Autodesk Inventor part; units mm, degrees
ref_plane "YZ Plane" through (0, 0, 0) normal (1, 0, 0) x (0, 1, 0)
ref_plane "XZ Plane" through (0, 0, 0) normal (0, 1, 0) x (-1, 0, 0)
ref_plane "XY Plane" through (0, 0, 0) normal (0, 0, 1) x (1, 0, 0)
sketch "Sketch1" plane through (0, 0, 0) normal (0, 0, 1) x (1, 0, 0)
  line L0 (4, 3.875) -> (-4, 3.875)
  line L1 (-4, 3.875) -> (-4, -3.875)
  line L2 (-4, -3.875) -> (4, -3.875)
  line L3 (4, -3.875) -> (4, 3.875)
  line L4 (4, 3.875) -> (-4, -3.875) construction
  line L5 (-4, 3.875) -> (4, -3.875) construction
  line L6 (4, 3.875) -> (9.5, 3.875)
  line L7 (-4, 3.875) -> (-9.5, 3.875)
  line L8 (4, -3.875) -> (9.5, 3.875)
  line L9 (-4, -3.875) -> (-9.5, 3.875)
  point P0 (0, 0)
  point P1 (0, 3.875)
  dimension "d0" = 8
  dimension "d1" = 7.75
  dimension "d2" = 9.5
  dimension "d3" = 9.5
extrude "Extrusion1" add sketch "Sketch1" along normal blind 25
sketch "Sketch2" plane through (-9.5, 3.875, 0) normal (0, 1, 0) x (1, 0, 0)
  line L0 (0, 0) -> (5.5, 0)
  line L1 (5.5, -25) -> (13.5, -25)
  line L2 (5.5, 0) -> (5.5, -25)
  line L3 (5.5, -25) -> (13.5, -25)
  line L4 (13.5, 0) -> (19, 0)
  line L5 (13.5, -25) -> (13.5, 0)
  line L6 (5.5, 0) -> (13.5, 0)
  line L7 (13.5, 0) -> (5.5, 0)
  point P0 (9.5, 0)
  dimension "d6" = 8
extrude "Extrusion2" add sketch "Sketch2" along normal blind 5
sketch "Sketch3" plane through (0, 0, 25) normal (0, 0, 1) x (1, 0, 0)
  line L0 (0, 0) -> (14.2258, 0)
  line L1 (-4, -3.875) -> (4, -3.875)
  line L2 (4, -3.875) -> (9.5, 3.875)
  line L3 (4, -3.875) -> (9.5, 3.875)
  line L4 (9.5, 3.875) -> (4, 3.875)
  line L5 (4, 3.875) -> (4, 8.875)
  line L6 (4, 3.875) -> (4, 8.875)
  line L7 (-4, 3.875) -> (-4, 8.875)
  line L8 (4, 8.875) -> (-4, 8.875)
  line L9 (-4, 8.875) -> (-4, 3.875)
  line L10 (-4, 3.875) -> (-9.5, 3.875)
  line L11 (-4, 3.875) -> (-9.5, 3.875)
  line L12 (-9.5, 3.875) -> (-4, -3.875)
  line L13 (42.75, -3.875) -> (48.25, 3.875)
  line L14 (48.25, 3.875) -> (42.75, 3.875)
  line L15 (42.75, 3.875) -> (42.75, 8.875)
  line L16 (42.75, 8.875) -> (34.75, 8.875)
  line L17 (34.75, 8.875) -> (34.75, 3.875)
  line L18 (34.75, 3.875) -> (29.25, 3.875)
  line L19 (29.25, 3.875) -> (34.75, -3.875)
  line L20 (34.75, -3.875) -> (42.75, -3.875)
  line L21 (34.75, 8.875) -> (42.75, 8.875)
  line L22 (42.75, 8.875) -> (42.75, 8.975)
  line L23 (42.75, 8.975) -> (34.75, 8.975)
  line L24 (34.75, 8.975) -> (34.75, 8.875)
  line L25 (4, 8.875) -> (-4, 8.875)
  line L26 (-4, 8.875) -> (-4, 8.975)
  line L27 (-4, 8.975) -> (4, 8.975)
  line L28 (4, 8.975) -> (4, 8.875)
  line L29 (-4, 8.975) -> (42.75, 8.975)
  line L30 (42.75, 8.975) -> (42.75, 10.675)
  line L31 (42.75, 10.675) -> (-4, 10.675)
  line L32 (-4, 10.675) -> (-4, 8.975)
  point P0 (6.75, 0)
  point P1 (38.75, 0)
  point P2 (52.9758, 0)
  point P3 (45.5, 0)
  dimension "d9" = 6.75
  dimension "d12" = 38.75
  dimension "d19" = 1.7
  dimension "d22" = 0.1
extrude "Extrusion3" add sketch "Sketch3" against normal blind 25 contours L26 L27 L28 L8 | L23 L22 L16 L24 | L16 L15 L14 L13 L20 L19 L18 L17
extrude "Extrusion4" add sketch "Sketch3" against normal blind 25 contours L32 L31 L30 L23 L29 L27
sketch "Sketch4" plane through (0, 0, 25) normal (0, 0, 1) x (1, 0, 0)
  line L0 (42.75, 10.675) -> (-4, 10.675)
  line L1 (-4, 10.675) -> (42.75, 10.675)
  line L2 (42.75, 10.675) -> (42.75, 92.475)
  line L3 (42.75, 92.475) -> (-4, 92.475)
  line L4 (-4, 92.475) -> (-4, 10.675)
  line L5 (-4, 10.675) -> (11, 10.675)
  line L6 (11, 10.675) -> (11, 92.475)
  line L7 (11, 92.475) -> (-4, 92.475)
  line L8 (-4, 92.475) -> (-4, 10.675)
  line L9 (78.9241, 46.475) -> (-27.5343, 46.475)
  line L10 (-27.5343, 46.475) -> (-27.5343, 66.675)
  line L11 (-27.5343, 66.675) -> (78.9241, 66.675)
  line L12 (78.9241, 66.675) -> (78.9241, 46.475)
  line L13 (4, 8.975) -> (34.75, 8.975)
  line L14 (-36.8215, 45.475) -> (107.9586, 45.475)
  line L15 (107.9586, 45.475) -> (107.9586, 29.475)
  line L16 (107.9586, 29.475) -> (-36.8215, 29.475)
  line L17 (-36.8215, 29.475) -> (-36.8215, 45.475)
  line L18 (-39.8107, 67.675) -> (114.95, 67.675)
  line L19 (114.95, 67.675) -> (114.95, 83.675)
  line L20 (114.95, 83.675) -> (-39.8107, 83.675)
  line L21 (-39.8107, 83.675) -> (-39.8107, 67.675)
  point P0 (0, 0)
  dimension "d23" = 81.8
  dimension "d24" = 15
  dimension "d25" = 37.5
  dimension "d26" = 20.2
  dimension "d27" = 16
  dimension "d28" = 18.8
  dimension "d29" = 16
  dimension "d30" = 1
  dimension "d31" = 1
  dimension "d36" = 8.8
  dimension "d37" = 47
extrude "Extrusion5" add sketch "Sketch4" against normal blind 25 contours L0 L4 L16 L6 | L16 L4 L14 L6 | L14 L4 L9 L6 | L9 L4 L11 L6 | L11 L4 L18 L6 | L18 L4 L20 L6 | L20 L4 L3 L6
sketch "Sketch5" plane through (0, 0, 25) normal (0, 0, 1) x (1, 0, 0)
  line L0 (11, 92.475) -> (11, 10.675)
  line L1 (42.75, 10.675) -> (42.75, 3.875)
  arc A0 (11, 16.49) -> (42.75, 10.675) centre (50.7681, 144.0402) ccw
  line L2 (11, 16.49) -> (11, 10.675)
  line L3 (11, 10.675) -> (42.75, 10.675)
  line L4 (42.75, 10.675) -> (11, 10.675)
  line L5 (34.75, 8.975) -> (4, 8.975)
  point P0 (0, 0)
extrude "Extrusion6" add sketch "Sketch5" against normal blind 25
sketch "Sketch6" plane through (-4, 3.875, 0) normal (-1, 0, 0) x (0, 0, 1)
  line L0 (25, 88.6) -> (0, 88.6)
  line L1 (25, 0) -> (25, 88.6)
  circle A0 centre (12.5, 71.8) radius 8.5
  circle A1 centre (12.5, 33.6) radius 8.5
  point P0 (0, -3.875)
  dimension "d38" = 16.8
  dimension "d39" = 12.5
  dimension "d40" = 17
  dimension "d41" = 55
  dimension "d42" = 17
extrude "Extrusion7" cut sketch "Sketch6" against normal blind 25
sketch "Sketch7" plane through (0, 0, 25) normal (0, 0, 1) x (1, 0, 0)
  line L0 (11, 16.49) -> (11, 92.475)
  line L1 (11, 92.475) -> (-4, 92.475)
  point P0 (0, 0)
  point P1 (3.5, 75.675)
  point P2 (3.5, 92.475)
  point P3 (3.5, 37.475)
  dimension "d45" = 7.5
  dimension "d46" = 16.8
  dimension "d47" = 55
hole "Hole1" at (3.5, 37.475, 25) at (3.5, 75.675, 25) direction (0, 0, -1) diameter 4 end through all
CAD build for the part. Positions are in the model's coordinates, mm. A direction names the side the tool comes from. Give positions to 0.01 mm unless a question says otherwise; leave off trailing zeros. Order: outer loops, then holes, each group sorted by start corner. A loop starts at its lowest first (then second) coordinate and runs counter-clockwise, first axis right, second up.
(1) Saw through at D-D, the plane y = 45. Give the cut face in (x, z).
(2) Saw through at C-C, the plane y = 81.5. Give the cut face in (x, z).
(3) Mould opens along Z. For faces 1 (the flat face through (9, 41, 25)), 2 (the cylindrical face through (3.395, 40.028, 20.607)), 3 (the flat face through (39, -3.875, 13)), 4 (the flat face through (9, 41, 0)) say: released by +Z, released by -Z, zero draft, split by the parting line, or undercut.
(4) Saw through at A-A, the plane z = 2.25. Give the cut face in (x, y) (3 decimals).
(5) Drill centre lines: L1, parallel to Y at x = 0, z = 12.5 (3 decimals); L2, parallel to Y at x = 3.5, z = 24.1 (3 decimals); L3, parallel to X at y = 5.5, z = 6.5. Where is each one in solid material? Low to high.
(6) Flat gauge pins, fed straight in: pin 1 (1.5 mm diameter, centred on y = 7.5, z = 14.5, fed in from -X); pin 2 (3 mm diameter, centred on x = 44.5, z = 13.5, fed in from +Y) (3 decimals); pin 3 (10 mm diameter, centred on y = 30.5, z = 19, fed in from +X); pin 4 (2.5 mm diameter, centred on x = 3.5, y = 37.475, fed in from -Z). Where does each tip first touch, or does it go through?
(7) Saw through at B-B, the plane z = 12.5. Give the cut face in (x, y) (3 decimals), then the cut area to 3 significant figures.
(8) Tool access for faces 5 (the flat face through (45.461, -0.054, 12.675)), 6 (the flat face through (-4, 49, 13)), 7 (the flat face through (6.711, -0.054, 12.325)), 8 (the flat face through (46, 3.875, 13)), 9 (the flat face through (32, 3.875, 13)): list every direction of +Z, -Z, +X, -X, +Y, -Y with a clear straight run to the whole face (end or side of a thin tool).
Results found:
1. outline: (-4, 0) - (11, 0) - (11, 8.55) - (-4, 8.55) - close; (-4, 16.45) - (11, 16.45) - (11, 25) - (-4, 25) - close
2. outline: (-4, 0) - (11, 0) - (11, 6.31) - (-4, 6.31) - close; (-4, 18.69) - (11, 18.69) - (11, 25) - (-4, 25) - close
3. face 1: released by +Z
3. face 2: undercut
3. face 3: zero draft
3. face 4: released by -Z
4. outline: (-9.5, 3.875) - (-4, -3.875) - (4, -3.875) - (9.5, 3.875) - (4, 3.875) - (4, 8.975) - (34.75, 8.975) - (34.75, 3.875) - (29.25, 3.875) - (34.75, -3.875) - (42.75, -3.875) - (48.25, 3.875) - (42.75, 3.875) - (42.75, 10.675) arc R133.609 cw to (11, 16.49) - (11, 92.475) - (-4, 92.475) - (-4, 3.875) - close; hole circle Ø4 at (3.5, 37.475); hole circle Ø4 at (3.5, 75.675)
5. L1: y = -3.875 to 28.975, 45.975 to 67.175, 84.175 to 92.475
5. L2: y = -3.875 to 35.475, 39.475 to 73.675, 77.675 to 92.475
5. L3: x = -4 to 4, 34.75 to 42.75
6. pin 1: stops at x = -4
6. pin 2: stops at y = 3.875
6. pin 3: stops at x = 11
6. pin 4: passes through
7. outline: (-9.5, 3.875) - (-4, -3.875) - (4, -3.875) - (9.5, 3.875) - (4, 3.875) - (4, 8.975) - (34.75, 8.975) - (34.75, 3.875) - (29.25, 3.875) - (34.75, -3.875) - (42.75, -3.875) - (48.25, 3.875) - (42.75, 3.875) - (42.75, 10.675) arc R133.609 cw to (11, 16.49) - (11, 28.975) - (-4, 28.975) - (-4, 3.875) - close; (-4, 45.975) - (11, 45.975) - (11, 67.175) - (-4, 67.175) - close; (-4, 84.175) - (11, 84.175) - (11, 92.475) - (-4, 92.475) - close
7. area: 1,160 mm2
8. face 5: +Z, -Z, +X, -Y
8. face 6: +Z, -Z, -X, +Y
8. face 7: +Z, -Z, -Y
8. face 8: +Z, -Z, +X, +Y
8. face 9: +Z, -Z
